from build123d import *

# Parameters (mm, degrees)
F1_DEPTH = 49.8911
F2_R     = 40.29989


with BuildPart() as f1:
    # F0 (on Right) → F1 (new body)
    with BuildSketch(Plane.YZ):
        Polygon((33.577301, 34.130178), (-24.453036, 3.655124), (-16.058711, -23.717679), (53.103238, -25.177559), (70.986792, 3.107668), align=None)
    extrude(amount=F1_DEPTH)

    # F2
    f2_edges = [f1.edges().sort_by_distance(p)[0] for p in [
        (24.94555, 53.103238, -25.177559),
    ]]
    fillet(f2_edges, radius=F2_R)


solid = f1.part
Part model, mm, in its own coordinate system. Give positions to 0.01 mm unless a question says otherwise; leave off trailing zeros. Loops run counter-clockwise (first coordinate to the right, second up) from the corner with the lowest first, then second, coordinate; pieces in that order, holes last.
(1) Pull direction Z, two halves, no side cores. Call faces 1 (the flat face through (24.596, 68.086, -1.481)), 2 (the flat face through (0, 23, -1)), 3 (the flat face through (24.596, 52.544, 18.402)): pulls with the +Z half, pulls with the -Z half, needs draft (parallel to the pull), parting line crosses it, or undercut.
Return value:
face 1: pulls with the -Z half
face 2: needs draft
face 3: pulls with the +Z half
(2) Pin check, flat tips, straight feed: pin 1 (2 mm diameter, centred on x = 22, z = 24, fed in from -Y); pin 2 (5 mm diameter, centred on x = 29.5, z = 14, fed in from +Y); pin 3 (4 mm diameter, centred on y = 32.5, z = -3, fed in from -X); pin 4 (2 mm diameter, centred on x = 17.5, y = -12.5, fed in from -Z). Stop position of each tip, or through.
Return value:
pin 1: stops at y = 12.38
pin 2: stops at y = 60.87
pin 3: stops at x = 0
pin 4: stops at z = -23.81
(3) Drill centre lines: line 1 along Y through (x, z) = (35, -19.5); line 2 along Z through (x, y) = (29, 4.5); line 3 along Z through (x, y) = (29.5, 8.5). Where is each one in solid material? Low to high.
Return value:
line 1: y = -17.35 to 51.01
line 2: z = -24.15 to 18.86
line 3: z = -24.24 to 20.96
(4) Band-saw the part on C-C (y = 43.5). Write the cut outline in (x, z).
Return value:
outline: (0, -22.78) - (49.89, -22.78) - (49.89, 25.9) - (0, 25.9) - close
(5) Band-saw the part on B-B (z = 21.5). Write the cut outline in (x, y).
Return value:
outline: (0, 9.53) - (49.89, 9.53) - (49.89, 48.81) - (0, 48.81) - close
(6) Band-saw the part on A-A (x = 10.5). Write the cut outline in (y, z).
Return value:
outline: (-24.45, 3.66) - (-16.06, -23.72) - (30.35, -24.7) arc R40.3 ccw to (65.26, -5.94) - (70.99, 3.11) - (33.58, 34.13) - close
